Here's how the part is built. I have some questions about the finished solid (model axes, mm). Face numbers are marked on the shaded views. Coordinates: 2 decimals unless noted, no trailing zeros. Write each loop counter-clockwise with the first axis right and the second up, starting at its lowest first coordinate (ties: lowest second). Pieces come first, ordered by that corner, then holes.
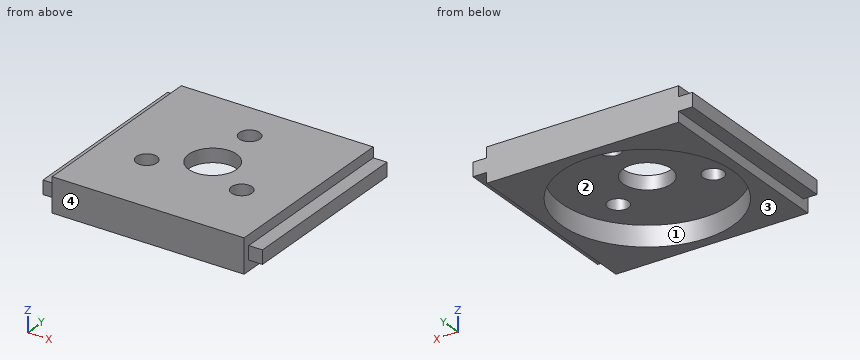
```python
from build123d import *

# Parameters (mm, degrees)
ESQUISSE1_W                  = 28
ESQUISSE1_H                  = 28
BOSS_EXTRU_1_DEPTH           = 5
ENL_V_MAT_EXTRU_1_DEPTH      = 40.912404087
ENL_V_MAT_EXTRU_1_DEPTH_BACK = 40.912404087
ESQUISSE2_R                  = 3.5
ESQUISSE3_W                  = 2
ESQUISSE3_H                  = 2
BOSS_EXTRU_2_DEPTH           = 27
ESQUISSE5_R                  = 1.5
ENL_V_MAT_EXTRU_3_DEPTH      = 42.340053217
ESQUISSE6_R                  = 12.5
ENL_V_MAT_EXTRU_4_DEPTH      = 3


with BuildPart() as part:
    # Esquisse1 → Boss.-Extru.1 (new body)
    with BuildSketch(Plane.XY):
        with Locations((14, 14)):
            Rectangle(ESQUISSE1_W, ESQUISSE1_H)
    extrude(amount=BOSS_EXTRU_1_DEPTH)

    # Esquisse2 → Enlèv. mat.-Extru.1 (cut, two sides: drawn at the far end of the back side and taken through both)
    with BuildSketch(Plane.XY.offset(5).offset(-ENL_V_MAT_EXTRU_1_DEPTH_BACK)):
        with Locations((14, 14)):
            Circle(ESQUISSE2_R)
    extrude(amount=ENL_V_MAT_EXTRU_1_DEPTH + ENL_V_MAT_EXTRU_1_DEPTH_BACK, mode=Mode.SUBTRACT)

    # Esquisse3 → Boss.-Extru.2 (add)
    with BuildSketch(Plane(origin=(0, 28, 0), x_dir=(1, 0, 0), z_dir=(0, 1, 0))):
        with Locations((-1, -2.5)):
            Rectangle(ESQUISSE3_W, ESQUISSE3_H)
        with Locations((29, -2.5)):
            Rectangle(ESQUISSE3_W, ESQUISSE3_H)
    extrude(amount=-BOSS_EXTRU_2_DEPTH)

    # Esquisse5 → Enlèv. mat.-Extru.3 (cut, through all)
    with BuildSketch(Plane(origin=(0, 0, 0), x_dir=(-1, 0, 0), z_dir=(0, 0, -1))):
        with Locations((-14, 22)):
            Circle(ESQUISSE5_R)
        with Locations((-20.92820323, 10)):
            Circle(ESQUISSE5_R)
        with Locations((-7.07179677, 10)):
            Circle(ESQUISSE5_R)
    extrude(amount=-ENL_V_MAT_EXTRU_3_DEPTH, mode=Mode.SUBTRACT)

    # Esquisse6 → Enlèv. mat.-Extru.4 (cut)
    with BuildSketch(Plane(origin=(0, 0, 0), x_dir=(-1, 0, 0), z_dir=(0, 0, -1))):
        with Locations((-14, 14)):
            Circle(ESQUISSE6_R)
    extrude(amount=-ENL_V_MAT_EXTRU_4_DEPTH, mode=Mode.SUBTRACT)


solid = part.part
```
1) Imagine slicing it at C-C on y = 15.5. Please give me the cut outline in (x, z).
Values follow:
outline: (-2, 1.5) - (0, 1.5) - (0, 0) - (1.59, 0) - (1.59, 3) - (10.84, 3) - (10.84, 5) - (0, 5) - (0, 3.5) - (-2, 3.5) - close; (17.16, 3) - (26.41, 3) - (26.41, 0) - (28, 0) - (28, 1.5) - (30, 1.5) - (30, 3.5) - (28, 3.5) - (28, 5) - (17.16, 5) - close
2) Imagine slicing it at D-D on z = 1.9. Please give me the cut outline in (x, y), then the cut area to 3 significant figures.
Values follow:
outline: (-2, 1) - (0, 1) - (0, 0) - (28, 0) - (28, 1) - (30, 1) - (30, 28) - (-2, 28) - close; hole circle Ø25 at (14, 14)
area: 401 mm2
3) We'd pull the mould along Y, two halves only. Please class the marked faces 1, 2, 3 and 4: pulls with the +Y half, pulls with the -Y half, needs draft (parallel to the pull), parting line crosses it, or undercut.
Values follow:
face 1: undercut
face 2: undercut
face 3: needs draft
face 4: pulls with the -Y half
4) I need wall thicknesses on probe 1 along Y at (x, z) = (14, 4.55); probe 2 along X at (y, z) = (14.25, 1.05); probe 3 along X at (y, z) = (14, 4.2). Which ranges of each line are inside material? Lowest first, please.
Values follow:
probe 1: y = 0 to 10.5, 17.5 to 20.5, 23.5 to 28
probe 2: x = 0 to 1.5, 26.5 to 28
probe 3: x = 0 to 10.5, 17.5 to 28
5) Imagine slicing it at A-A on z = 4.2. Please give me the cut outline in (x, y).
Values follow:
outline: (0, 0) - (28, 0) - (28, 28) - (0, 28) - close; hole circle Ø3 at (7.07, 10); hole circle Ø7 at (14, 14); hole circle Ø3 at (14, 22); hole circle Ø3 at (20.93, 10)
6) Will these pins go through, and if not, where does the flat tip stop? pin 1 (2.5 mm diameter, centred on x = 20.93, y = 10, fed in from +Z); pin 2 (2 mm diameter, centred on x = -1.5, y = 15.5, fed in from -Z); pin 3 (2 mm diameter, centred on x = 28.5, z = 2.5, fed in from -Y); pin 4 (4 mm diameter, centred on x = 14, y = 22, fed in from -Z).
Values follow:
pin 1: passes through
pin 2: stops at z = 1.5
pin 3: stops at y = 0
pin 4: stops at z = 3
7) Imagine slicing it at B-B on x = 14. Please give me the cut outline in (y, z), then the cut area to 3 significant figures.
Values follow:
outline: (0, 0) - (1.5, 0) - (1.5, 3) - (10.5, 3) - (10.5, 5) - (0, 5) - close; (17.5, 3) - (20.5, 3) - (20.5, 5) - (17.5, 5) - close; (23.5, 3) - (26.5, 3) - (26.5, 0) - (28, 0) - (28, 5) - (23.5, 5) - close
area: 45.0 mm2
